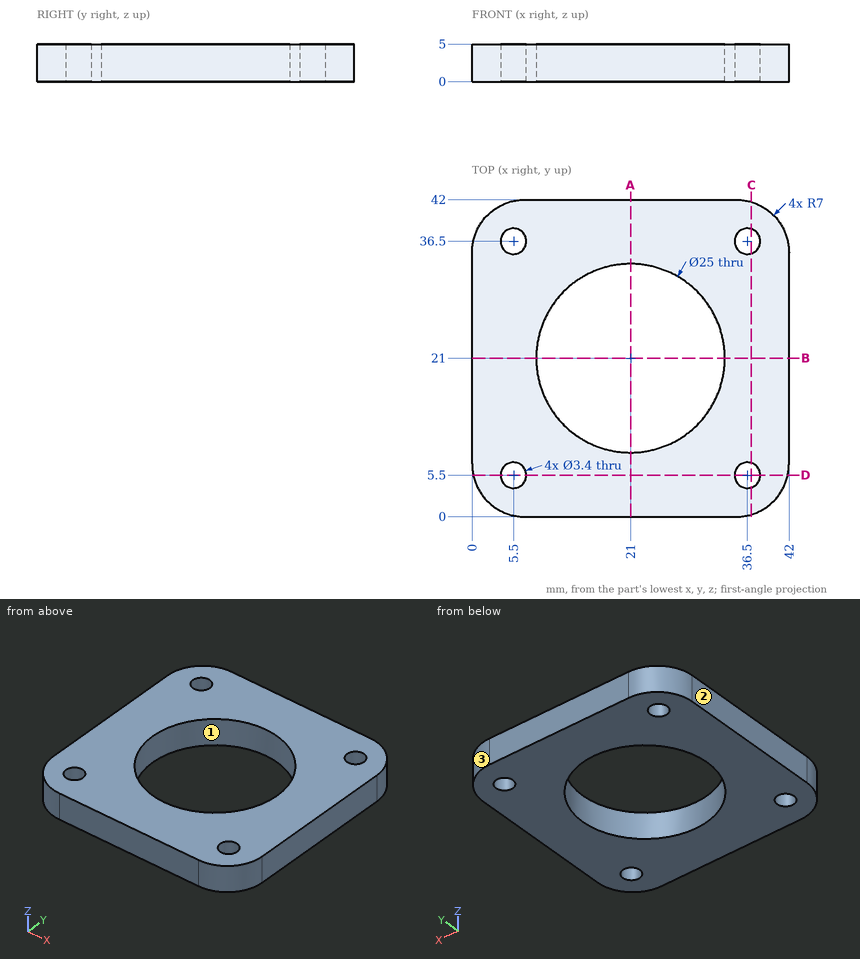
For this review, use the dimensioned drawing (mm, ordinates from the lowest corner) and the shaded views. Give positions to 0.01 mm unless a question says otherwise; leave off trailing zeros. Loops run counter-clockwise (first coordinate to the right, second up) from the corner with the lowest first, then second, coordinate; pieces in that order, holes last.
Item 1: Draft analysis for pull direction Y (two halves, no side actions). For the marked faces 1, 2 and 3, state which applies: +Y half, -Y half, draft (parallel to the pull), parting line (faces both ways), or undercut.
Item 2: Take a section at C-C, the plane x = 37. State the section outline as (y, z) points, and give its area (3 significant figures).
Item 3: For line 1 along Y through (x, z) = (5.5, 2.75); line 2 along X through (y, z) = (38, 4.5); line 3 along X through (y, z) = (24, 0.8), list the stretches that pass through material, from the lowest coordinate up.
Item 4: Insertion check: pin 1 (1 mm diameter, centred on x = 22.5, z = 2.5, fed in from -Y). The pin has a flat end and moves straight along its axis. Give the tip position at first contact, or say it passes through.
Item 5: Take a section at A-A, the plane x = 21. State the section outline as (y, z) points, and give its area (3 significant figures).
Item 6: Take a section at D-D, the plane y = 5.5. State the section outline as (x, z) points.
Calculated:
1. face 1: undercut
1. face 2: draft
1. face 3: +Y half
2. outline: (0.29, 0) - (3.88, 0) - (3.88, 5) - (0.29, 5) - close; (7.12, 0) - (34.88, 0) - (34.88, 5) - (7.12, 5) - close; (38.12, 0) - (41.71, 0) - (41.71, 5) - (38.12, 5) - close
2. area: 175 mm2
3. line 1: y = 0.16 to 3.8, 7.2 to 34.8, 38.2 to 41.84
3. line 2: x = 0.68 to 4.7, 6.3 to 35.7, 37.3 to 41.32
3. line 3: x = 0 to 8.87, 33.13 to 42
4. pin 1: stops at y = 0
5. outline: (0, 0) - (8.5, 0) - (8.5, 5) - (0, 5) - close; (33.5, 0) - (42, 0) - (42, 5) - (33.5, 5) - close
5. area: 85.0 mm2
6. outline: (0.16, 0) - (3.8, 0) - (3.8, 5) - (0.16, 5) - close; (7.2, 0) - (34.8, 0) - (34.8, 5) - (7.2, 5) - close; (38.2, 0) - (41.84, 0) - (41.84, 5) - (38.2, 5) - close
